Geometry: final body of the model. Coordinates: model frame, mm. A direction names the side the tool comes from. Coordinates: 2 decimals unless noted, no trailing zeros. Write each loop counter-clockwise with the first axis right and the second up, starting at its lowest first coordinate (ties: lowest second). Pieces come first, ordered by that corner, then holes. Notation, with made-up numbers: (-33, 56.5) - (15, 56.5) arc R20 cw to (15, 92.5) - close; hole circle Ø8 at (25, 0.25). An arc over 180 degrees is marked (long way). Put each result on its own line as item: value.
```python
from build123d import *

# Parameters (mm, degrees)
SKETCH2_W            = 22.5
SKETCH2_H            = 23
BOSS_EXTRUDE1_DEPTH  = 12
SKETCH19_W           = 12
SKETCH19_H           = 2.48
BOSS_EXTRUDE8_DEPTH  = 4.82
SKETCH20_W           = 12
SKETCH20_H           = 2.48
BOSS_EXTRUDE9_DEPTH  = 4.82
SKETCH21_R           = 2.4
BOSS_EXTRUDE10_DEPTH = 4.4
SKETCH21_3_R         = 2.4
SKETCH21_3_R_2       = 0.95
BOSS_EXTRUDE11_DEPTH = 7.27
CUT_EXTRUDE5_DEPTH   = 2.49


with BuildPart() as part:
    # Sketch2 → Boss-Extrude1 (new body)
    with BuildSketch(Plane(origin=(0, 0, 0), x_dir=(0, 0, -1), z_dir=(1, 0, 0))):
        Rectangle(SKETCH2_W, SKETCH2_H)
    extrude(amount=BOSS_EXTRUDE1_DEPTH)

    # Sketch19 → Boss-Extrude8 (add)
    with BuildSketch(Plane.XY.offset(11.25)):
        with Locations((6, 6.24)):
            Rectangle(SKETCH19_W, SKETCH19_H)
    extrude(amount=BOSS_EXTRUDE8_DEPTH)

    # Sketch20 → Boss-Extrude9 (add)
    with BuildSketch(Plane(origin=(0, 0, -11.25), x_dir=(-1, 0, 0), z_dir=(0, 0, -1))):
        with Locations((-6, 6.24)):
            Rectangle(SKETCH20_W, SKETCH20_H)
    extrude(amount=BOSS_EXTRUDE9_DEPTH)

    # Sketch21 → Boss-Extrude10 (add)
    # profile 1 of 6: a face of its own
    with BuildSketch(Plane(origin=(0, 11.5, 0), x_dir=(1, 0, 0), z_dir=(0, 1, 0))):
        with BuildLine():
            ThreePointArc((6, 11.25), (1.757359316, 9.49264069), (0, 5.250000008))
            ThreePointArc((0, 5.250000008), (0.861906966, 2.151613326), (3.2, -0.056599665))
            Line((3.2, -0.056599665), (3.287216195, -0.056599665))
            ThreePointArc((3.287216195, -0.056599665), (6, 2.05), (8.712783805, -0.056599665))
            Line((8.712783805, -0.056599665), (8.8, -0.056599665))
            ThreePointArc((8.8, -0.056599665), (11.138093031, 2.151613323), (12, 5.25))
            ThreePointArc((12, 5.25), (10.242640687, 9.492640687), (6, 11.25))
        make_face()
        with Locations(Location((6, 5.25, 0), (0, 0, 90))):
            Circle(SKETCH21_R, mode=Mode.SUBTRACT)
    # profile 2 of 6: a face of its own
    with BuildSketch(Plane(origin=(0, 11.5, 0), x_dir=(1, 0, 0), z_dir=(0, 1, 0))):
        with BuildLine():
            Line((6, -0.75), (8.8, -0.75))
            ThreePointArc((8.8, -0.75), (8.780610633, -0.421055467), (8.722711067, -0.096666667))
            ThreePointArc((8.722711067, -0.096666667), (7.4, -0.584380858), (6, -0.75))
        make_face()
    # profile 3 of 6: a face of its own
    with BuildSketch(Plane(origin=(0, 11.5, 0), x_dir=(1, 0, 0), z_dir=(0, 1, 0))):
        with BuildLine():
            ThreePointArc((3.277288933, -0.096666667), (3.219389367, -0.421055467), (3.2, -0.75))
            Line((3.2, -0.75), (6, -0.75))
            ThreePointArc((6, -0.75), (4.6, -0.584380858), (3.277288933, -0.096666667))
        make_face()
    # profile 4 of 6: a face of its own
    with BuildSketch(Plane(origin=(0, 11.5, 0), x_dir=(1, 0, 0), z_dir=(0, 1, 0))):
        with BuildLine():
            ThreePointArc((3.2, -0.75), (4.020101013, -2.729898987), (6, -3.55))
            ThreePointArc((6, -3.55), (7.979898987, -2.729898987), (8.8, -0.75))
            Line((8.8, -0.75), (6, -0.75))
            Line((6, -0.75), (3.2, -0.75))
        make_face()
    # profile 5 of 6: a face of its own
    with BuildSketch(Plane(origin=(0, 11.5, 0), x_dir=(1, 0, 0), z_dir=(0, 1, 0))):
        with BuildLine():
            ThreePointArc((8.712783805, -0.056599665), (6, 2.05), (3.287216195, -0.056599665))
            Line((3.287216195, -0.056599665), (8.712783805, -0.056599665))
        make_face()
    # profile 6 of 6: a face of its own
    with BuildSketch(Plane(origin=(0, 11.5, 0), x_dir=(1, 0, 0), z_dir=(0, 1, 0))):
        with BuildLine():
            ThreePointArc((3.277288933, -0.096666667), (4.6, -0.584380858), (6, -0.75))
            ThreePointArc((6, -0.75), (7.4, -0.584380858), (8.722711067, -0.096666667))
            ThreePointArc((8.722711067, -0.096666667), (8.717821272, -0.076614872), (8.712783805, -0.056599665))
            Line((8.712783805, -0.056599665), (3.287216195, -0.056599665))
            ThreePointArc((3.287216195, -0.056599665), (3.282178728, -0.076614872), (3.277288933, -0.096666667))
        make_face()
    extrude(amount=BOSS_EXTRUDE10_DEPTH)

    # Sketch21<3> → Boss-Extrude11 (add)
    with BuildSketch(Plane(origin=(0, 11.5, 0), x_dir=(1, 0, 0), z_dir=(0, 1, 0))):
        with Locations(Location((6, 5.25, 0), (0, 0, 90))):
            Circle(SKETCH21_3_R)
        with Locations(Location((6, 5.25, 0), (0, 0, 90))):
            Circle(SKETCH21_3_R_2, mode=Mode.SUBTRACT)
    extrude(amount=BOSS_EXTRUDE11_DEPTH)

    # Sketch23 → Cut-Extrude5 (cut)
    with BuildSketch(Plane(origin=(0, 7.48, 0), x_dir=(1, 0, 0), z_dir=(0, 1, 0))):
        with BuildLine():
            Line((6.65, -15.248541033), (6.65, -16.07))
            Line((6.65, -16.07), (5.35, -16.07))
            Line((5.35, -16.07), (5.35, -15.248541033))
            ThreePointArc((5.35, -15.248541033), (6, -11.77), (6.65, -15.248541033))
        make_face()
    cut_extrude5 = extrude(amount=-CUT_EXTRUDE5_DEPTH, mode=Mode.SUBTRACT)

    # Mirror3: Cut-Extrude5 across plane
    add(cut_extrude5.mirror(Plane.XY), mode=Mode.SUBTRACT)


solid = part.part
```
1. Pin query (flat end, axial travel): pin 1 Ø3.5 at (x, y) = (4.5, -0.5) entering from +Z; pin 2 Ø6 at (x, y) = (5, -1) entering from -Z; pin 3 Ø2 at (x, z) = (10.5, 6) entering from +Y. Return the tip coordinate at first contact, or that it passes through.
Answer below:
pin 1: stops at z = 11.25
pin 2: stops at z = -11.25
pin 3: stops at y = 11.5
2. Section query D-D (z = -8.5). Return loops of the section in (x, y).
Answer below:
outline: (0, -11.5) - (12, -11.5) - (12, 11.5) - (11.04, 11.5) - (11.04, 15.9) - (0.96, 15.9) - (0.96, 11.5) - (0, 11.5) - close
3. Mould query, pull axis Z, two halves, no side actions, for faces 4 (the flat face through (9, 6, 16.07)), 5 (the cylindrical face through (5.93, 6.26, -11.77)), 6 (the flat face through (11, 11.5, -10)), 7 (the cylindrical face through (6.84, 15.08, -5.69)). Classes: +Z half, -Z half, draft (parallel to the pull), parting line (faces both ways), or undercut.
Answer below:
face 4: +Z half
face 5: undercut
face 6: draft
face 7: undercut
4. Ray query, probe 1 along X at (y, z) = (6.3, -13.57); probe 2 along Y at (x, z) = (1.5, -11.5); probe 3 along Z at (x, y) = (6, 8). Return the intervals inside material, ascending. Write a range as from..to.
Answer below:
probe 1: x = 0..4.2, 7.8..12
probe 2: y = 5..7.48
probe 3: z = -11.25..11.25
5. Section query C-C (y = 1). Return loops of the section in (x, z).
Answer below:
outline: (0, -11.25) - (12, -11.25) - (12, 11.25) - (0, 11.25) - close
6. Section query A-A (z = 13.57). Return loops of the section in (x, y), then the cut area to 3 significant figures.
Answer below:
outline: (0, 5) - (4.2, 5) - (4.2, 7.48) - (0, 7.48) - close; (7.8, 5) - (12, 5) - (12, 7.48) - (7.8, 7.48) - close
area: 20.8 mm²
7. Section query B-B (z = 3). Return loops of the section in (x, y), then the cut area to 3 significant figures.
Answer below:
outline: (0, -11.5) - (12, -11.5) - (12, 11.5) - (7.67, 11.5) - (7.67, 15.9) - (4.33, 15.9) - (4.33, 11.5) - (0, 11.5) - close
area: 291 mm²
8. Set-up query: faces 1 (the flat face through (4.6, 7.48, 12)), 2 (the flat face through (6, -3, 11.25)), 3 (the flat face through (7.4, 7.48, -12)). Return all of +Z, -Z, +X, -X, +Y, -Y with unobstructed straight access to the full face (end or side cutting, diameter ignored); none if empty.
Answer below:
face 1: +Z, +X, -X, +Y
face 2: +Z, +X, -X, -Y
face 3: -Z, +X, -X, +Y
